Verification items for the finished model (mm, model axes). A direction names the side the tool comes from. Give positions to 0.01 mm unless a question says otherwise; leave off trailing zeros. Order: outer loops, then holes, each group sorted by start corner. A loop starts at its lowest first (then second) coordinate and runs counter-clockwise, first axis right, second up. Notation, with made-up numbers: M -15.5,-36 L 29.5,-36 A38 cw 29.5,2 Z; hole C 65.5,0 d6. An arc over 180 degrees is marked long. Answer as a JSON object with one key per item and string values.
```python
from build123d import *

# Parameters (mm, degrees)
ESQUISSE1_R                  = 11.75
BOSS_EXTRU_1_DEPTH           = 0.0001
ESQUISSE2_W                  = 40
ESQUISSE2_H                  = 40
BOSS_EXTRU_2_DEPTH           = 5
ENL_V_MAT_EXTRU_1_DEPTH      = 3.5
ESQUISSE4_R                  = 1.75
ENL_V_MAT_EXTRU_2_DEPTH      = 2
ESQUISSE5_W                  = 2
ESQUISSE5_H                  = 40
ESQUISSE5_W_2                = 8
BOSS_EXTRU_3_DEPTH           = 7
ESQUISSE6_W                  = 2
ESQUISSE6_H                  = 40
BOSS_EXTRU_4_DEPTH           = 14
ENL_V_MAT_EXTRU_3_DEPTH      = 14
ENL_V_MAT_EXTRU_3_DEPTH_BACK = 14
ESQUISSE7_R                  = 1
CONG_1_R                     = 2
CONG_2_R                     = 1.5
CONG_3_R                     = 1.5
ESQUISSE10_W                 = 8
ESQUISSE10_H                 = 31
ENL_V_MAT_EXTRU_4_DEPTH      = 10
CONG_4_R                     = 2
ESQUISSE11_W                 = 20.8
ESQUISSE11_H                 = 22
ENL_V_MAT_EXTRU_5_DEPTH      = 10
CONG_5_R                     = 2
ESQUISSE12_W                 = 4
ESQUISSE12_H                 = 5
BOSS_EXTRU_5_DEPTH           = 10


with BuildPart() as part:
    # Esquisse1 → Boss.-Extru.1 (new body)
    with BuildSketch(Plane(origin=(0, 0, 0), x_dir=(1, 0, 0), z_dir=(0, 1, 0))):
        with Locations(Location((0, 0, 0), (0, 0, 270))):
            Circle(ESQUISSE1_R)
    extrude(amount=BOSS_EXTRU_1_DEPTH)

    # Esquisse2 → Boss.-Extru.2 (add)
    with BuildSketch(Plane(origin=(0, 0.0001, 0), x_dir=(1, 0, 0), z_dir=(0, 1, 0))):
        Rectangle(ESQUISSE2_W, ESQUISSE2_H)
    extrude(amount=BOSS_EXTRU_2_DEPTH)

    # Esquisse3 → Enlèv. mat.-Extru.1 (cut)
    with BuildSketch(Plane(origin=(0, 5.0001, 0), x_dir=(1, 0, 0), z_dir=(0, 1, 0))):
        Polygon((-13.825684219, 12.6), (-12.151368439, 15.5), (-13.825684219, 18.4), (-17.174315781, 18.4), (-18.848631561, 15.5), (-17.174315781, 12.6), align=None)
        Polygon((-18.848631561, -15.5), (-17.174315781, -18.4), (-13.825684219, -18.4), (-12.151368439, -15.5), (-13.825684219, -12.6), (-17.174315781, -12.6), align=None)
        Polygon((12.151368439, -15.5), (13.825684219, -18.4), (17.174315781, -18.4), (18.848631561, -15.5), (17.174315781, -12.6), (13.825684219, -12.6), align=None)
        Polygon((13.825684219, 12.6), (17.174315781, 12.6), (18.848631561, 15.5), (17.174315781, 18.4), (13.825684219, 18.4), (12.151368439, 15.5), align=None)
    extrude(amount=-ENL_V_MAT_EXTRU_1_DEPTH, mode=Mode.SUBTRACT)

    # Esquisse4 → Enlèv. mat.-Extru.2 (cut)
    with BuildSketch(Plane(origin=(0, 1.5001, 0), x_dir=(1, 0, 0), z_dir=(0, 1, 0))):
        with Locations(Location((-15.5, 15.5, 0), (0, 0, 270))):
            Circle(ESQUISSE4_R)
        with Locations(Location((15.5, 15.5, 0), (0, 0, 270))):
            Circle(ESQUISSE4_R)
        with Locations(Location((-15.5, -15.5, 0), (0, 0, 270))):
            Circle(ESQUISSE4_R)
        with Locations(Location((15.5, -15.5, 0), (0, 0, 270))):
            Circle(ESQUISSE4_R)
    extrude(amount=-ENL_V_MAT_EXTRU_2_DEPTH, mode=Mode.SUBTRACT)

    # Esquisse5 → Boss.-Extru.3 (add)
    with BuildSketch(Plane(origin=(0, 5.0001, 0), x_dir=(1, 0, 0), z_dir=(0, 1, 0))):
        with Locations((11, 0)):
            Rectangle(ESQUISSE5_W, ESQUISSE5_H)
        with Locations((0.9, 0)):
            Rectangle(ESQUISSE5_W_2, ESQUISSE5_H)
    extrude(amount=BOSS_EXTRU_3_DEPTH)

    # Esquisse6 → Boss.-Extru.4 (add)
    with BuildSketch(Plane(origin=(0, 12.0001, 0), x_dir=(1, 0, 0), z_dir=(0, 1, 0))):
        with Locations((-2.1, 0)):
            Rectangle(ESQUISSE6_W, ESQUISSE6_H)
    extrude(amount=BOSS_EXTRU_4_DEPTH)

    # Esquisse7 → Enlèv. mat.-Extru.3 (cut, two sides: drawn at the far end of the back side and taken through both)
    with BuildSketch(Plane(origin=(-1.1, 0, 0), x_dir=(0, 0, -1), z_dir=(1, 0, 0)).offset(-ENL_V_MAT_EXTRU_3_DEPTH_BACK)):
        with Locations(Location((-13.5, 20.0001, 0), (0, 0, 180))):
            Circle(ESQUISSE7_R)
        with Locations(Location((13.5, 20.0001, 0), (0, 0, 180))):
            Circle(ESQUISSE7_R)
        Polygon((0, 26.0001), (-11.6, 26.0001), (-11.6, 5.0001), (11.6, 5.0001), (11.6, 26.0001), align=None)
    extrude(amount=ENL_V_MAT_EXTRU_3_DEPTH + ENL_V_MAT_EXTRU_3_DEPTH_BACK, mode=Mode.SUBTRACT)

    # Congé1
    cong_1_edges = [part.edges().sort_by_distance(p)[0] for p in [
        (-2.1, 26.0001, 20),
        (-2.1, 26.0001, -20),
        (-2.1, 26.0001, 11.6),
        (-2.1, 26.0001, -11.6),
    ]]
    fillet(cong_1_edges, radius=CONG_1_R)

    # Congé2
    cong_2_edges = [part.edges().sort_by_distance(p)[0] for p in [
        (4.9, 8.5001, 20),
        (4.9, 8.5001, -20),
        (4.9, 8.5001, -11.6),
        (4.9, 8.5001, 11.6),
    ]]
    fillet(cong_2_edges, radius=CONG_2_R)

    # Congé3
    cong_3_edges = [part.edges().sort_by_distance(p)[0] for p in [
        (20, 2.5001, 20),
        (20, 2.5001, -20),
        (-20, 2.5001, -20),
        (-20, 2.5001, 20),
    ]]
    fillet(cong_3_edges, radius=CONG_3_R)

    # Esquisse10 → Enlèv. mat.-Extru.4 (cut)
    with BuildSketch(Plane(origin=(0, 5.0001, 0), x_dir=(1, 0, 0), z_dir=(0, 1, 0))):
        with Locations((16, -4.5)):
            Rectangle(ESQUISSE10_W, ESQUISSE10_H)
    extrude(amount=-ENL_V_MAT_EXTRU_4_DEPTH, mode=Mode.SUBTRACT)

    # Congé4
    cong_4_edges = [part.edges().sort_by_distance(p)[0] for p in [
        (20, 2.5001, -11),
    ]]
    fillet(cong_4_edges, radius=CONG_4_R)

    # Esquisse11 → Enlèv. mat.-Extru.5 (cut)
    with BuildSketch(Plane(origin=(0, 5.0001, 0), x_dir=(1, 0, 0), z_dir=(0, 1, 0))):
        with Locations((-5.6, 0)):
            Rectangle(ESQUISSE11_W, ESQUISSE11_H)
    extrude(amount=-ENL_V_MAT_EXTRU_5_DEPTH, mode=Mode.SUBTRACT)

    # Congé5
    # the kernel refuses this fillet: 2 mm, written as the material it adds along each edge
    with BuildSketch(Plane(origin=(4.8, 5.0001, 11), x_dir=(0, 0, -1), z_dir=(0, -1, 0))) as cong_5_piece_1_section:
        with BuildLine():
            CenterArc((CONG_5_R, -CONG_5_R), CONG_5_R, 90, 90)
            Line((0, -CONG_5_R), (0, 0))
            Line((0, 0), (CONG_5_R, 0))
        make_face()
    cong_5_piece_1 = extrude(amount=10, mode=Mode.PRIVATE)
    cong_5_piece_1 = split(cong_5_piece_1, bisect_by=Plane(origin=(4.313925052, 0, 10.490530882), z_dir=(0, 1, 0)), keep=Keep.TOP, mode=Mode.PRIVATE)
    add(cong_5_piece_1)
    with BuildSketch(Plane(origin=(-16, 5.0001, 11), x_dir=(0, 0, -1), z_dir=(0, -1, 0))) as cong_5_piece_2:
        with BuildLine():
            CenterArc((CONG_5_R, CONG_5_R), CONG_5_R, 180, 90)
            Line((0, CONG_5_R), (0, 0))
            Line((0, 0), (CONG_5_R, 0))
        make_face()
    extrude(amount=5)
    with BuildSketch(Plane(origin=(4.8, 5.0001, -11), x_dir=(-1, 0, 0), z_dir=(0, -1, 0))) as cong_5_piece_3_section:
        with BuildLine():
            CenterArc((CONG_5_R, -CONG_5_R), CONG_5_R, 90, 90)
            Line((0, -CONG_5_R), (0, 0))
            Line((0, 0), (CONG_5_R, 0))
        make_face()
    cong_5_piece_3 = extrude(amount=10, mode=Mode.PRIVATE)
    cong_5_piece_3 = split(cong_5_piece_3, bisect_by=Plane(origin=(4.313925052, 0, -10.490530882), z_dir=(0, 1, 0)), keep=Keep.TOP, mode=Mode.PRIVATE)
    add(cong_5_piece_3)
    with BuildSketch(Plane(origin=(-16, 5.0001, -11), x_dir=(0, 0, 1), z_dir=(0, -1, 0))) as cong_5_piece_4:
        with BuildLine():
            CenterArc((CONG_5_R, -CONG_5_R), CONG_5_R, 90, 90)
            Line((0, -CONG_5_R), (0, 0))
            Line((0, 0), (CONG_5_R, 0))
        make_face()
    extrude(amount=5)

    # Esquisse12 → Boss.-Extru.5 (add)
    with BuildSketch(Plane(origin=(0, 5.0001, 0), x_dir=(1, 0, 0), z_dir=(0, 1, 0))):
        with Locations((-18, 0)):
            Rectangle(ESQUISSE12_W, ESQUISSE12_H)
    extrude(amount=BOSS_EXTRU_5_DEPTH)


solid = part.part
```
Q1. Section check C-C on y = 12.5. Record the cut outline in (x, z).
Resolved:
{"outline": "M -20,-2.5 L -16,-2.5 L -16,2.5 L -20,2.5 Z; M -3.1,-20 L -1.1,-20 L -1.1,-11.6 L -3.1,-11.6 Z; M -3.1,11.6 L -1.1,11.6 L -1.1,20 L -3.1,20 Z"}
Q2. Tool access check on faces 1 (the face through (-18, 3.27, -16.97)), 2 (the face through (-6, 3, -11)), 3 (the face through (4.45, 8.55, 19.57)), 4 (the face through (2, 12, 16)). Record the directions out of +Z, -Z, +X, -X, +Y, -Y that give a thin tool (end or side, any length) a straight path to the whole face; none if there is none.
Resolved:
{"face 1": "+Y", "face 2": "+Y, -Y", "face 3": "+Z, +Y", "face 4": "+Z, -Z, +X, +Y"}
Q3. Section check A-A on x = 15.5. Record the cut outline in (y, z).
Resolved:
{"outline": "M 0,-20 L 5,-20 L 5,-18.4 L 1.5,-18.4 L 1.5,-17.25 L 0,-17.25 Z; M 0,-13.75 L 1.5,-13.75 L 1.5,-12.6 L 5,-12.6 L 5,-11 L 0,-11 Z"}
Q4. Section check B-B on y = 8. Record the cut outline in (x, z).
Resolved:
{"outline": "M -20,-2.5 L -16,-2.5 L -16,2.5 L -20,2.5 Z; M -3.1,-20 L 3.4,-20 A1.5 ccw 4.9,-18.5 L 4.9,-13.1 A1.5 ccw 3.4,-11.6 L -3.1,-11.6 Z; M -3.1,11.6 L 3.4,11.6 A1.5 ccw 4.9,13.1 L 4.9,18.5 A1.5 ccw 3.4,20 L -3.1,20 Z; M 10,-20 L 12,-20 L 12,-11.6 L 10,-11.6 Z; M 10,11.6 L 12,11.6 L 12,20 L 10,20 Z"}
Q5. Gauge pin test, flat ends, axial feed: pin 1 Ø2 at (x, z) = (10.5, -16) entering from +Y; pin 2 Ø2.5 at (y, z) = (22, 17.5) entering from +X; pin 3 Ø4.5 at (x, z) = (16.5, -15) entering from +Y. Record the tip position at first contact, or that the pin passes through.
Resolved:
{"pin 1": "stops at y = 12", "pin 2": "stops at x = -1.1", "pin 3": "stops at y = 5"}
Q6. Release check for a two-part mould opening along X. For faces 5 (the face through (12, 8, -16)), 6 (the face through (4.45, 8.55, -19.57)), 7 (the face through (11, 9, 11.6)) record: +X half, -X half, draft (parallel to the pull), parting line (faces both ways), or undercut.
Resolved:
{"face 5": "+X half", "face 6": "undercut", "face 7": "draft"}
Q7. Section check D-D on x = -15.5. Record the cut outline in (y, z).
Resolved:
{"outline": "M 0,-20 L 5,-20 L 5,-18.4 L 1.5,-18.4 L 1.5,-17.25 L 0,-17.25 Z; M 0,-13.75 L 1.5,-13.75 L 1.5,-12.6 L 5,-12.6 L 5,-10.32 L 0,-10.32 Z; M 0,10.32 L 5,10.32 L 5,12.6 L 1.5,12.6 L 1.5,13.75 L 0,13.75 Z; M 0,17.25 L 1.5,17.25 L 1.5,18.4 L 5,18.4 L 5,20 L 0,20 Z"}
Q8. Material ranges on L1, parallel to X at y = 0.8, z = -15.5; L2, parallel to Z at x = 1.5, y = 2.5; L3, parallel to Z at x = -2, y = 9.25, recorded low to high.
Resolved:
{"L1": "x = -20 to -17.25, -13.75 to 13.75, 17.25 to 20", "L2": "z = -20 to -11, 11 to 20", "L3": "z = -20 to -11.6, 11.6 to 20"}
